```python
from build123d import *

# Parameters (mm, degrees)
F0_R     = 3.175
F1_DEPTH = 36.83


# Not quite as in the source:
# - a length typed as a fraction of an inch, garbled in the dataset ("3 / 203.2 mm" for 3/8 in), is restored
# - a feature names something its author has since deleted; it is built from what else it names


with BuildPart() as f1:
    # F0 (on Right) → F1 (new body)
    with BuildSketch(Plane.YZ):
        Circle(F0_R)
    extrude(amount=-F1_DEPTH)

    # F2 (on Front) → F3 (revolve)
    with BuildSketch(Plane.XZ):
        with BuildLine():
            Line((0, 3.175), (0, 0))
            Line((0, 0), (5.715, 0))
            ThreePointArc((5.715, 0), (4.0411152545, 4.0411152545), (0, 5.715))
            Line((0, 5.715), (0, 3.175))
        make_face()
    revolve(axis=Axis((0, 0, 0), (1, 0, 0)))

    # F4: F1 across face


with BuildPart() as f1_1:
    add(f1.part)
    add(f1.part.mirror(Plane(origin=(-36.83, 0, 0), x_dir=(0, 1, 0), z_dir=(-1, 0, 0))))


solid = f1_1.part
```
Geometry: final body of the model. Coordinates: model frame, mm. Coordinates: 2 decimals unless noted, no trailing zeros. Order: outer loops, then holes, each group sorted by start corner. A loop starts at its lowest first (then second) coordinate and runs counter-clockwise, first axis right, second up. Notation, with made-up numbers: M 45,-20 L 92,-20 A8 cw 92,-9 Z; hole C 64.25,37 d1. An arc over 180 degrees is marked long. Answer as CSV lines item,"result".
Q1. Line query: probe 1 along X at (y, z) = (-4.25, 2.25); probe 2 along X at (y, z) = (-3.75, -3.5); probe 3 along Z at (x, y) = (-13, 1.75). Output: solid intervals per line, ascending. Write a range as [from, to].
Answers:
probe 1,"x = [-76.75, -73.66], [0, 3.09]"
probe 2,"x = [-76.18, -73.66], [0, 2.52]"
probe 3,"z = [-2.65, 2.65]"
Q2. Section C-C on x = -45. Return the cut outline in (y, z) (3 decimals).
Answers:
outline,"C 0,0 d6.35"
Q3. Section A-A on z = 0. Return the cut outline in (x, y) (3 decimals), and give its area (3 significant figures).
Answers:
outline,"M -73.66,-5.715 L -73.66,-3.175 L 0,-3.175 L 0,-5.715 A5.715 ccw 0,5.715 L 0,3.175 L -73.66,3.175 L -73.66,5.715 A5.715 ccw Z"
area,"570 mm^2"
Q4. First-contact query: P1, Ø6, axis at x = -48, z = 2.5, coming from the -Y side (3 decimals); P2, Ø1, axis at x = -9.5, z = 1.5, coming from the +Y side; P3, Ø6, axis at x = -6.5, y = -2.5, coming from the -Z side (3 decimals). Flat tips, straight axial feed; report the tip coordinate or a pass-through.
Answers:
P1,"stops at y = -3.175"
P2,"stops at y = 3.01"
P3,"stops at z = -3.175"
